Design review of the part built by this model. Coordinates are the model's own, in mm. Face numbers are marked on the shaded views. A direction names the side the tool comes from. Round coordinates to 2 decimals unless told otherwise and drop trailing zeros. Order: outer loops, then holes, each group sorted by start corner. A loop starts at its lowest first (then second) coordinate and runs counter-clockwise, first axis right, second up. Notation, with made-up numbers: M -11,0 L 28,0 A21 ccw 28,32 Z; hole C 31.5,45.5 d5. An arc over 180 degrees is marked long. Write item = value, one per line. Start each with the question number.
Autodesk Inventor part; units mm, degrees
ref_plane "작업 평면1" through (-13, 15, 0) normal (0, 1, 0) x (1, 0, 0)
ref_plane "작업 평면2" through (0, -5, 10) normal (1, 0, 0) x (0, 0, -1)
ref_plane "YZ Plane" through (0, 0, 0) normal (1, 0, 0) x (0, 1, 0)
sketch "스케치1" plane through (0, 0, 0) normal (0, 0, 1) x (1, 0, 0)
  line L0 (-13, -5) -> (13, -5)
  line L1 (13, -5) -> (13, 5)
  line L2 (13, 5) -> (-13, 5)
  line L3 (-13, 5) -> (-13, -5)
  line L4 (-13, -5) -> (13, 5) construction
  line L5 (13, -5) -> (-13, 5) construction
  circle A0 centre (0, 0) radius 2.5
  dimension "d0" = 26
  dimension "d1" = 10
  dimension "d2" = 5
extrude "돌출1" add sketch "스케치1" along normal blind 10
sketch "스케치2" plane through (-13, 5, 0) normal (0, 1, 0) x (1, 0, 0)
  line L0 (26, 0) -> (0, 0)
  line L1 (26, -10) -> (0, -10)
  line L2 (0, 0) -> (5, 0)
  line L3 (5, 0) -> (5, -10)
  line L4 (5, -10) -> (0, -10)
  line L5 (0, -10) -> (0, 0)
  line L6 (13, 0) -> (13, -10)
  line L7 (26, 0) -> (21, 0)
  line L8 (21, 0) -> (21, -10)
  line L9 (21, -10) -> (26, -10)
  line L10 (26, -10) -> (26, 0)
  point P0 (0, -10)
  point P1 (21, 0)
  dimension "d5" = 5
  dimension "d6" = 8
extrude "돌출2" add sketch "스케치2" along normal blind 10 contours L10 L1 L8 L0 | L3 L1 L5 L0
sketch "스케치3" plane through (-13, 5, 0) normal (-1, 0, 0) x (0, 0, 1)
  circle A0 centre (5, 5) radius 2.5
  line L0 (0, 10) -> (10, 10)
  line L1 (10, -10) -> (10, 10)
  point P0 (0, -5)
  point P1 (10, 0)
  point P2 (10, 5)
  point P3 (5, 10)
  point P4 (5, 10)
  dimension "d9" = 5
extrude "돌출3" cut sketch "스케치3" against normal through all
ref_plane "작업 평면1" through (-13, 15, 0) normal (0, 1, 0) x (1, 0, 0)
mirror "미러1" about plane through (-10.5, 15, 5) normal (0, 1, 0) of "돌출3", "돌출2"
sketch "스케치4" plane through (0, 0, 0) normal (0, 0, -1) x (-1, 0, 0)
  line L0 (-13, 5) -> (-13, 25)
  line L1 (13, -5) -> (-13, -5)
  line L2 (-13, 25) -> (13, 25)
  line L3 (13, 25) -> (13, -5)
  line L4 (13, -5) -> (-13, -5)
  line L5 (-13, -5) -> (-13, 25)
  point P0 (0, 0)
  point P1 (13, 25)
extrude "돌출4" add sketch "스케치4" along normal blind 5
ref_plane "작업 평면2" through (0, -5, 10) normal (1, 0, 0) x (0, 0, -1)
sketch "스케치5" plane through (0, -5, 10) normal (1, 0, 0) x (0, 0, -1)
  line L0 (10, 10) -> (10, 30)
  line L1 (10, 30) -> (15, 30)
  line L2 (15, 30) -> (15, 35)
  line L3 (15, 35) -> (10, 35)
  line L4 (10, 35) -> (10, 30)
  circle A0 centre (12.5, 32.5) radius 1.5
  point P0 (10, 5)
  point P1 (10, 32.5)
  point P2 (12.5, 35)
  dimension "d16" = 5
  dimension "d19" = 3
extrude "돌출5" add sketch "스케치5" along normal mid plane 15
extrude "돌출6" cut sketch "스케치5" along normal mid plane 5
fillet "모깎기2" radius 2.5 4 edges at (-5, 30, -5) (-5, 30, 0) (5, 30, -5) (5, 30, 0)
properties part number "SteeringFrame"
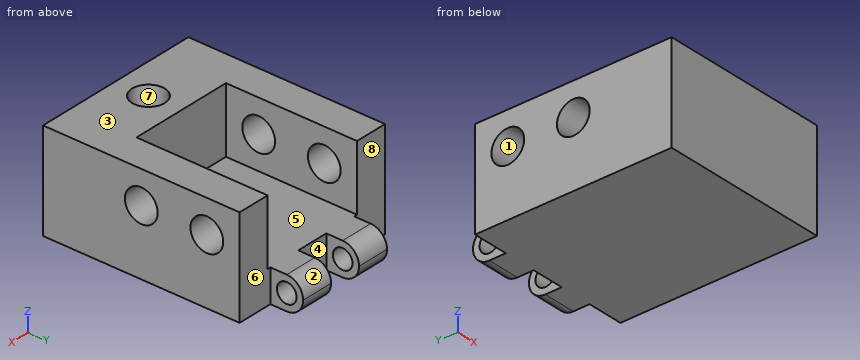
(1) Consider section D-D, the plane y = 0. Write out the cut boundary in (x, z), then the cut area to 3 significant figures.
(2) For line 1 along X through (y, z) = (15.5, 8); line 2 along Y through (x, z) = (0, 5.25); line 3 along Y through (x, z) = (-6, -2.5), list the stretches that pass through material, from the lowest coordinate up. Write a range as [from, to].
(3) Draft analysis for pull direction Y (two halves, no side actions). For the marked faces 1, 2 and 3, state which applies: pulls with the +Y half, pulls with the -Y half, needs draft (parallel to the pull), parting line crosses it, or undercut.
(4) Insertion check: pin 1 (3 mm diameter, centred on x = 0, y = 0, fed in from +Z); pin 2 (3.5 mm diameter, centred on y = 27.5, z = -2.5, fed in from -X); pin 3 (1.6 mm diameter, centred on x = 11, z = 2.5, fed in from +Y). Each pin has a flat end and moves straight along its axis. Give the tip position at first contact, or say it passes through.
(5) Consider section C-C, the plane z = 4.25. Write out the cut boundary in (x, y), then the cut area to 3 significant figures.
(6) For the marked faces 4, 5, 6, 7 and 8, list the 3-axis set-ups (+Z, -Z, +X, -X, +Y, -Y) from which the entire face can be reached by the end or side of a thin tool; tool diameter is ignored.
(7) Consider section A-A, the plane y = 22. Write out the cut boundary in (x, z), then the cut area to 3 significant figures.
Completed:
q1.outline = M -13,-5 L 13,-5 L 13,10 L 2.5,10 L 2.5,0 L -2.5,0 L -2.5,10 L -13,10 Z
q1.area = 340 mm2
q2.line_1 = [-13, -8], [8, 13]
q2.line_2 = [-5, -2.5], [2.5, 5]
q2.line_3 = [-5, 26], [29, 30]
q3.face_1 = undercut
q3.face_2 = pulls with the +Y half
q3.face_3 = needs draft
q4.pin_1 = 0
q4.pin_2 = -7.5
q4.pin_3 = 25
q5.outline = M -13,-5 L 13,-5 L 13,7.62 L 8,7.62 L 8,5 L -8,5 L -8,7.62 L -13,7.62 Z; M -13,12.38 L -8,12.38 L -8,17.62 L -13,17.62 Z; M -13,22.38 L -8,22.38 L -8,25 L -13,25 Z; M 8,12.38 L 13,12.38 L 13,17.62 L 8,17.62 Z; M 8,22.38 L 13,22.38 L 13,25 L 8,25 Z; hole C 0,0 d5
q5.area = 345 mm2
q6.face_4 = +Z, -Z, +Y
q6.face_5 = +Z, +Y
q6.face_6 = +Z, -Z, +X, +Y
q6.face_7 = +Z
q6.face_8 = +Z, -Z, -X, +Y
q7.outline = M -13,-5 L 13,-5 L 13,3.5 L 8,3.5 L 8,0 L -8,0 L -8,3.5 L -13,3.5 Z; M -13,6.5 L -8,6.5 L -8,10 L -13,10 Z; M 8,6.5 L 13,6.5 L 13,10 L 8,10 Z
q7.area = 200 mm2
